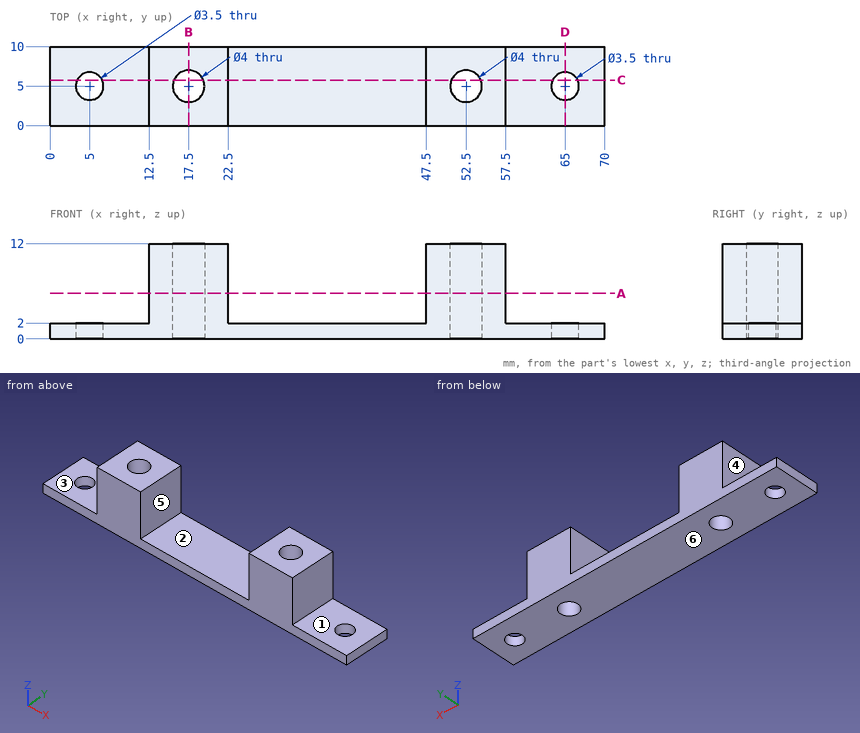
The figure shows three views and two pictorial views of one solid part (mm, origin at its lowest corner). Answer the questions. A direction names the side the tool comes from. Give positions to 0.01 mm unless a question says otherwise; leave off trailing zeros. Write each loop counter-clockwise with the first axis right and the second up, starting at its lowest first coordinate (ties: lowest second). Pieces come first, ordered by that corner, then holes.
Q1. For a pull along X with two mould halves and no side action, classify the marked faces 4, 5 and 6 as released by +X, released by -X, zero draft, split by the parting line, or undercut.
Answer:
face 4: released by -X
face 5: undercut
face 6: zero draft
Q2. The part is cut by section A-A on z = 5.75. Give the vertices of the cut face in (x, y), and give its area (3 significant figures).
Answer:
outline: (12.5, 0) - (22.5, 0) - (22.5, 10) - (12.5, 10) - close; (47.5, 0) - (57.5, 0) - (57.5, 10) - (47.5, 10) - close; hole circle Ø4 at (17.5, 5); hole circle Ø4 at (52.5, 5)
area: 175 mm2
Q3. Given pin 1 (3 mm diameter, centred on x = 36.5, z = 4, fed in from +Y); pin 2 (3 mm diameter, centred on y = 4, z = 8, fed in from -X); pin 3 (5 mm diameter, centred on x = 40, y = 2.5, fed in from +Z), each flat-ended and moving along its own axis, determine where each tip first touches the part or whether it passes through.
Answer:
pin 1: passes through
pin 2: stops at x = 12.5
pin 3: stops at z = 2
Q4. Straight lines are drawn through the part: L1, parallel to Y at x = 65, z = 0.9; L2, parallel to X at y = 3.5, z = 8; L3, parallel to Y at x = 52.5, z = 8.75. For each, find the intervals that lie inside material, in ascending order.
Answer:
L1: y = 0 to 3.25, 6.75 to 10
L2: x = 12.5 to 16.18, 18.82 to 22.5, 47.5 to 51.18, 53.82 to 57.5
L3: y = 0 to 3, 7 to 10
Q5. The part is cut by section C-C on y = 5.75. Give the vertices of the cut face in (x, z), and give its area (3 significant figures).
Answer:
outline: (0, 0) - (3.42, 0) - (3.42, 2) - (0, 2) - close; (6.58, 0) - (15.65, 0) - (15.65, 12) - (12.5, 12) - (12.5, 2) - (6.58, 2) - close; (19.35, 0) - (50.65, 0) - (50.65, 12) - (47.5, 12) - (47.5, 2) - (22.5, 2) - (22.5, 12) - (19.35, 12) - close; (54.35, 0) - (63.42, 0) - (63.42, 2) - (57.5, 2) - (57.5, 12) - (54.35, 12) - close; (66.58, 0) - (70, 0) - (70, 2) - (66.58, 2) - close
area: 238 mm2
Q6. The part is cut by section D-D on x = 65. Give the vertices of the cut face in (y, z), and give its area (3 significant figures).
Answer:
outline: (0, 0) - (3.25, 0) - (3.25, 2) - (0, 2) - close; (6.75, 0) - (10, 0) - (10, 2) - (6.75, 2) - close
area: 13.0 mm2
Q7. The part is cut by section B-B on x = 17.5. Give the vertices of the cut face in (y, z), and give its area (3 significant figures).
Answer:
outline: (0, 0) - (3, 0) - (3, 12) - (0, 12) - close; (7, 0) - (10, 0) - (10, 12) - (7, 12) - close
area: 72.0 mm2
Q8. A tool of negligible diameter and unlimited length cuts with its end or side. For the marked faces 1, 2 and 3, from which of +Z, -Z, +X, -X, +Y, -Y can it reach the whole face along a straight path? Write none if from no direction.
Answer:
face 1: +Z, +X, +Y, -Y
face 2: +Z, +Y, -Y
face 3: +Z, -X, +Y, -Y
